Answer from the drawing. Dimensions are ordinates in mm from the lowest x, y and z of the part. Give positions to 0.01 mm unless a question says otherwise; leave off trailing zeros. Loops run counter-clockwise (first coordinate to the right, second up) from the corner with the lowest first, then second, coordinate; pieces in that order, holes last. Notation, with made-up numbers: (71, 0) - (101, 0) arc R28 cw to (101, 30) - close; hole circle Ø7 at (44.5, 47.5). An arc over 180 degrees is marked (long way). One line per question, with ' | ' between items. Start each with the question number.
1. Each of these flat-tipped pins is pushed along its axis until it touches: pin 1 (1 mm diameter, centred on y = 2, z = 8, fed in from +X) (1 decimal); pin 2 (1.5 mm diameter, centred on x = 4, y = 1.5, fed in from +Z) (1 decimal); pin 3 (3 mm diameter, centred on x = 6.35, z = 6.35, fed in from -Y); pin 4 (2 mm diameter, centred on y = 2, z = 1.5, fed in from +X). Where does it stop, or does it pass through?
2. Find the intervals of material crossed by line 1 (X direction, y = 2.25, z = 6.35); line 2 (Z direction, x = 6.75, y = 1.15); line 3 (Z direction, x = 8.5, y = 2.15) (1 decimal), in increasing order.
3. For a pull along Z with two mould halves and no side action, classify the marked faces 1, 2 and 3 as released by +Z, released by -Z, zero draft, split by the parting line, or undercut.
4. Section C-C (y = 2.45) is taken. Determine the outline of the cut face in (x, z), plus the area to 3 significant figures.
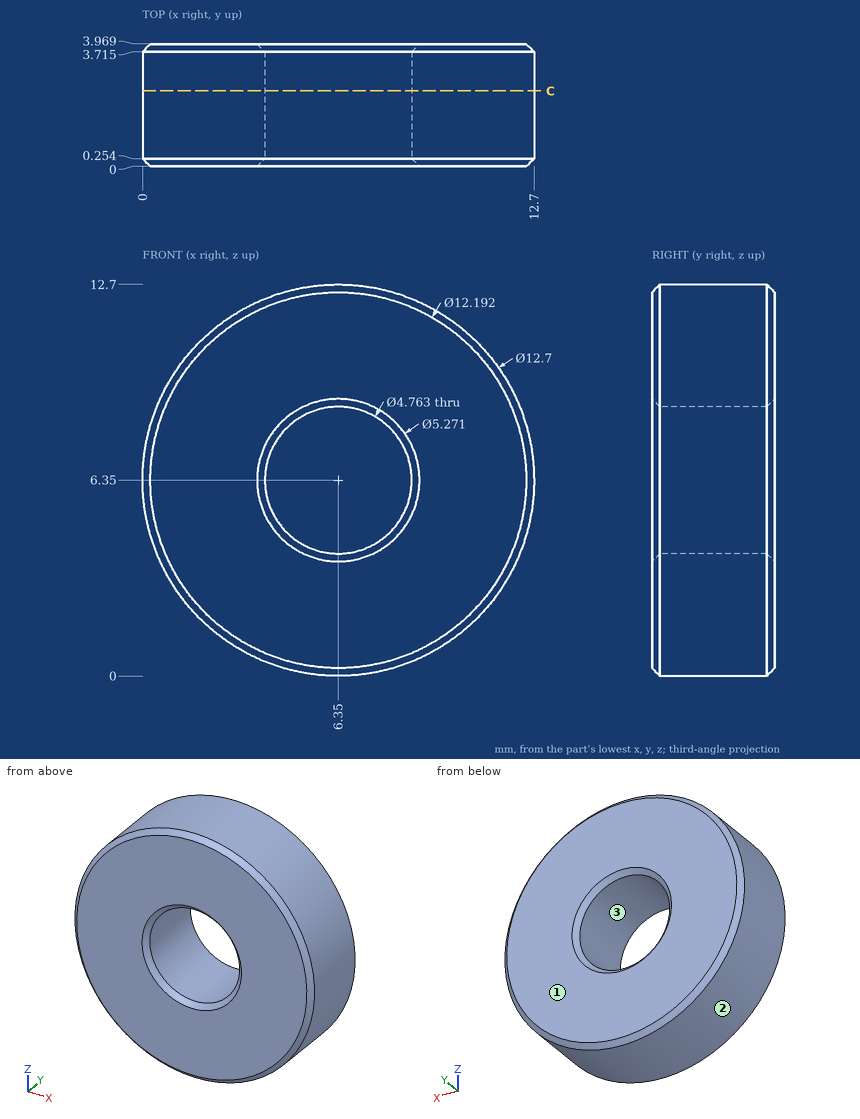
Conclusion:
1) pin 1: x = 12.6 | pin 2: z = 12.5 | pin 3: through | pin 4: x = 11.4
2) line 1: 0 to 3.97, 8.73 to 12.7 | line 2: 0.01 to 4, 8.7 to 12.69 | line 3: 0.4 to 5.3, 7.4 to 12.3
3) face 1: zero draft | face 2: split by the parting line | face 3: undercut
4) outline: circle Ø12.7 at (6.35, 6.35); hole circle Ø4.76 at (6.35, 6.35) | area: 109 mm²
